from build123d import *

# Parameters (mm, degrees)
F2_DEPTH  = 1.27
F5_R      = 3.048
F6_DEPTH  = 1.8034
F7_SIZE   = 0.2
F8_R      = 0.635
F9_DEPTH  = 2.54
F11_DEPTH = 3.048
F12_R     = 3.302
F13_DEPTH = 11.43


with BuildPart() as f2:
    # F1 (on Top) → F2 (new body)
    with BuildSketch(Plane.XY):
        Polygon((3.9624, 2.2876927066), (0, 4.5753854133), (-3.9624, 2.2876927066), (-3.9624, -2.2876927066), (0, -4.5753854133), (3.9624, -2.2876927066), align=None)
    extrude(amount=F2_DEPTH)

    # F3 (on Right) → F4 (revolve, cut)
    with BuildSketch(Plane.YZ):
        with BuildLine():
            ThreePointArc((3.8753854133, 1.27), (4.3703601601, 1.0649747468), (4.5753854133, 0.57))
            Line((4.5753854133, 0.57), (4.5753854133, 1.27))
            Line((4.5753854133, 1.27), (3.8753854133, 1.27))
        make_face()
    revolve(axis=Axis((0, 0, -1.1243047193), (0, 0, 1)), mode=Mode.SUBTRACT)

    # F5 (on face) → F6 (join)
    with BuildSketch(Plane.XY.offset(1.27)):
        Circle(F5_R)
    extrude(amount=F6_DEPTH)

    # F7
    f7_edges = [f2.edges().sort_by_distance(p)[0] for p in [
        (-3.048, 0, 3.0734),
    ]]
    chamfer(f7_edges, length=F7_SIZE)

    # F8 (on face) → F9 (join)
    with BuildSketch(Plane.XY.offset(3.0734)):
        Circle(F8_R)
    extrude(amount=F9_DEPTH)

    # F10 (on face) → F11 (cut)
    with BuildSketch(Plane.XY.offset(5.6134)):
        with BuildLine():
            Line((-0.635, 0), (-0.4572, 0))
            ThreePointArc((-0.4572, 0), (0, -0.4572), (0.4572, 0))
            Line((0.4572, 0), (0.635, 0))
            ThreePointArc((0.635, 0), (0, 0.635), (-0.635, 0))
        make_face()
    extrude(amount=-F11_DEPTH, mode=Mode.SUBTRACT)

    # F12 (on face) → F13 (join)
    with BuildSketch(Plane(origin=(0, 0, 0), x_dir=(1, 0, 0), z_dir=(0, 0, -1))):
        Circle(F12_R)
    extrude(amount=F13_DEPTH)


solid = f2.part
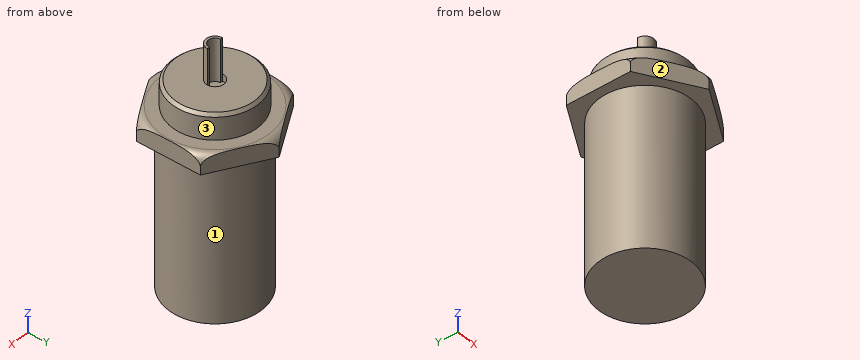
Design review of the part built by this model. Coordinates are the model's own, in mm. Face numbers are marked on the shaded views. A direction names the side the tool comes from. Give positions to 0.01 mm unless a question says otherwise; leave off trailing zeros. Loops run counter-clockwise (first coordinate to the right, second up) from the corner with the lowest first, then second, coordinate; pieces in that order, holes last. Notation, with made-up numbers: (78, 25) -> (132, 25) arc R13 ccw to (132, 36) -> close; hole circle Ø10 at (-3, 20.25). An arc over 180 degrees is marked (long way). One line per question, with ' | ' between items. Start each with the question number.
(1) We need section A-A (z = -2). State the section outline as (x, y) points, and give its area (3 significant figures).
(2) Insertion check: P1, Ø1, axis at x = -2, z = 0, coming from the -Y side; P2, Ø2, axis at y = 3, z = -8, coming from the +X side. Each pin has a flat end and moves straight along its axis. Give the tip position at first contact, or say it passes through.
(3) For the marked faces 1, 2 and 3, list the 3-axis set-ups (+Z, -Z, +X, -X, +Y, -Y) from which the entire face can be reached by the end or side of a thin tool; tool diameter is ignored.
(4) For line 1 (Z direction, x = 2.75, y = 2); line 2 (Z direction, x = -2.75, y = 0.5); line 3 (X direction, y = 3, z = -6.75), list the stretches that pass through material, from the lowest coordinate up.
(5) We need section B-B (z = 2.25). State the section outline as (x, y) points.
The answers:
1) outline: circle Ø6.6 at (0, 0) | area: 34.3 mm^2
2) P1: stops at y = -3.71 | P2: stops at x = 2.63
3) face 1: -Z | face 2: +Z, -Z, -X, -Y | face 3: +Z
4) line 1: z = 0 to 1.27 | line 2: z = -11.43 to 3.07 | line 3: x = -1.38 to 1.38
5) outline: circle Ø6.1 at (0, 0)
